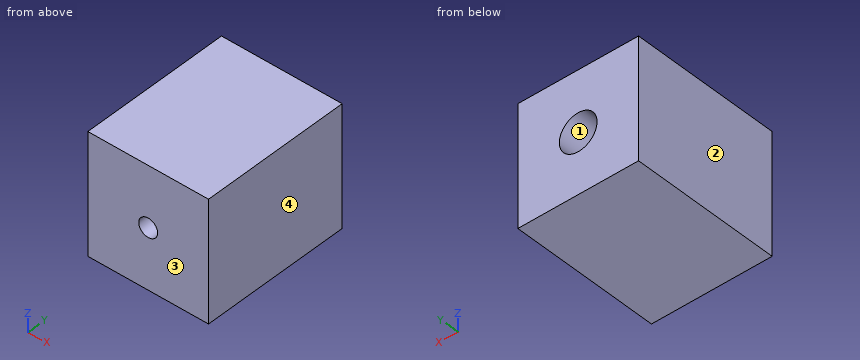
from build123d import *

# Parameters (mm, degrees)
SKETCH_1_R          = 6
EXTRUDE_1_DEPTH     = 40
SKETCH_2_R          = 5
CUT_EXTRUDE_2_DEPTH = 30
SKETCH_3_R          = 2.5
CUT_EXTRUDE_4_DEPTH = 10
SKETCH_5_R          = 16
SKETCH_5_R_2        = 6
EXTRUDE_1_2_DEPTH   = 40
SKETCH_6_W          = 32
SKETCH_6_H          = 32
SKETCH_6_W_2        = 12
SKETCH_6_H_2        = 12
EXTRUDE_2_DEPTH     = 40


with BuildPart() as part:
    # 草圖1 → Extrude 1 (new body)
    with BuildSketch(Plane(origin=(0, 0, 0), x_dir=(1, 0, 0), z_dir=(0, 1, 0))):
        with Locations(Location((0, 0, 0), (0, 0, 270))):
            Circle(SKETCH_1_R)
    extrude(amount=EXTRUDE_1_DEPTH)

    # 草圖2 → 除料-伸長2 (cut)
    with BuildSketch(Plane(origin=(0, 40, 0), x_dir=(1, 0, 0), z_dir=(0, 1, 0))):
        with Locations(Location((0, 0, 0), (0, 0, 270))):
            Circle(SKETCH_2_R)
    extrude(amount=-CUT_EXTRUDE_2_DEPTH, mode=Mode.SUBTRACT)

    # 草圖3 → 除料-伸長4 (cut)
    with BuildSketch(Plane.XZ):
        with Locations(Location((0, 0, 0), (0, 0, 270))):
            Circle(SKETCH_3_R)
    extrude(amount=-CUT_EXTRUDE_4_DEPTH, mode=Mode.SUBTRACT)

    # 草圖5 → Extrude 1 2 (add)
    with BuildSketch(Plane(origin=(0, 0, 0), x_dir=(1, 0, 0), z_dir=(0, 1, 0))):
        Circle(SKETCH_5_R)
        Circle(SKETCH_5_R_2, mode=Mode.SUBTRACT)
    extrude(amount=EXTRUDE_1_2_DEPTH)

    # 草圖6 → 伸長-薄件2 (add)
    with BuildSketch(Plane(origin=(0, 40, 0), x_dir=(1, 0, 0), z_dir=(0, 1, 0))):
        Rectangle(SKETCH_6_W, SKETCH_6_H)
        Rectangle(SKETCH_6_W_2, SKETCH_6_H_2, mode=Mode.SUBTRACT)
    extrude(amount=-EXTRUDE_2_DEPTH)


solid = part.part
Geometry: final body of the model. Coordinates: model frame, mm. Face numbers are marked on the shaded views. Give positions to 0.01 mm unless a question says otherwise; leave off trailing zeros. Loops run counter-clockwise (first coordinate to the right, second up) from the corner with the lowest first, then second, coordinate; pieces in that order, holes last. Notation, with made-up numbers: (-3, 13.5) -> (10, 13.5) arc R19 cw to (10, 28.5) -> close; hole circle Ø11 at (7.5, 46.5). An arc over 180 degrees is marked (long way). Put each result on its own line as item: value.
1. Cut plane C-C (y = 5.5). Return the cut outline in (x, z), plus the area to 3 significant figures.
Taken from the geometry:
outline: (-16, -16) -> (16, -16) -> (16, 16) -> (-16, 16) -> close; hole circle Ø5 at (0, 0)
area: 1,000 mm2
2. Ray query, line 1 along X through (y, z) = (21, 0); line 2 along X through (y, z) = (5.5, 0); line 3 along Z through (x, y) = (2, 24.5). Return the intervals inside material, ascending. Write a range as [from, to].
Taken from the geometry:
line 1: x = [-16, -5], [5, 16]
line 2: x = [-16, -2.5], [2.5, 16]
line 3: z = [-16, -4.58], [4.58, 16]
3. Cut plane D-D (y = 16.5). Return the cut outline in (x, z), plus the area to 3 significant figures.
Taken from the geometry:
outline: (-16, -16) -> (16, -16) -> (16, 16) -> (-16, 16) -> close; hole circle Ø10 at (0, 0)
area: 945 mm2
4. Pin query (flat end, axial travel): P1, Ø3, axis at x = 6, z = 10.5, coming from the -Y side; P2, Ø5, axis at x = 0.5, z = 0, coming from the +Y side. Return the tip coordinate at first contact, or that it passes through.
Taken from the geometry:
P1: stops at y = 0
P2: stops at y = 10
5. Cut plane A-A (x = 0). Return the cut outline in (y, z), plus the area to 3 significant figures.
Taken from the geometry:
outline: (0, -16) -> (40, -16) -> (40, -5) -> (10, -5) -> (10, -2.5) -> (0, -2.5) -> close; (0, 2.5) -> (10, 2.5) -> (10, 5) -> (40, 5) -> (40, 16) -> (0, 16) -> close
area: 930 mm2
6. Pull-direction query (X, two-part tool) for the marked faces 1, 2, 3 and 4; classes: released by +X, released by -X, zero draft, split by the parting line, or undercut.
Taken from the geometry:
face 1: undercut
face 2: released by -X
face 3: zero draft
face 4: released by +X
7. Cut plane B-B (z = 0). Return the cut outline in (x, y).
Taken from the geometry:
outline: (-16, 0) -> (-2.5, 0) -> (-2.5, 10) -> (-5, 10) -> (-5, 40) -> (-16, 40) -> close; (2.5, 0) -> (16, 0) -> (16, 40) -> (5, 40) -> (5, 10) -> (2.5, 10) -> close
